from build123d import *

# Parameters (mm, degrees)
SKETCH1_R           = 12.2
BOSS_EXTRUDE1_DEPTH = 23.5
SKETCH2_R           = 12.5
BOSS_EXTRUDE2_DEPTH = 27
SKETCH3_R           = 3.5
BOSS_EXTRUDE3_DEPTH = 1.5
SKETCH4_R           = 2
BOSS_EXTRUDE4_DEPTH = 11


with BuildPart() as part:
    # Sketch1 → Boss-Extrude1 (new body, symmetric)
    with BuildSketch(Plane(origin=(0, 0, 0), x_dir=(1, 0, 0), z_dir=(0, 1, 0))):
        Circle(SKETCH1_R)
    extrude(amount=BOSS_EXTRUDE1_DEPTH, both=True)

    # Sketch2 → Boss-Extrude2 (add)
    with BuildSketch(Plane(origin=(0, 23.5, 0), x_dir=(1, 0, 0), z_dir=(0, 1, 0))):
        Circle(SKETCH2_R)
    extrude(amount=BOSS_EXTRUDE2_DEPTH)

    # Sketch3 → Boss-Extrude3 (add)
    with BuildSketch(Plane(origin=(0, 50.5, 0), x_dir=(1, 0, 0), z_dir=(0, 1, 0))):
        Circle(SKETCH3_R)
    extrude(amount=BOSS_EXTRUDE3_DEPTH)

    # Sketch4 → Boss-Extrude4 (add)
    with BuildSketch(Plane(origin=(0, 52, 0), x_dir=(1, 0, 0), z_dir=(0, 1, 0))):
        Circle(SKETCH4_R)
    extrude(amount=BOSS_EXTRUDE4_DEPTH)


solid = part.part
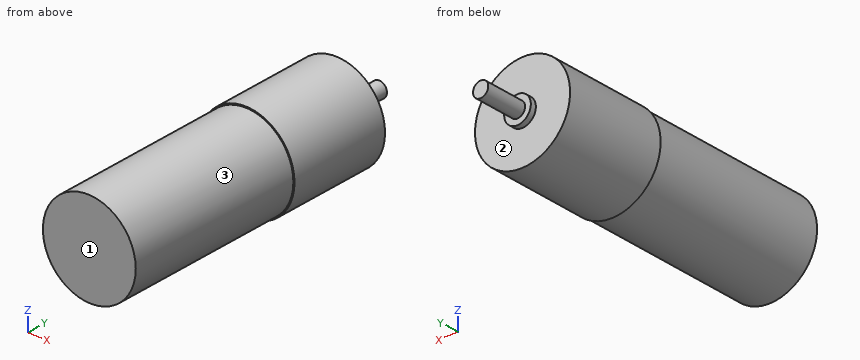
Geometry check sheet. Reference: the model listing, model coordinates, mm. Face numbers are marked on the shaded views. A direction names the side the tool comes from. Coordinates: 2 decimals unless noted, no trailing zeros. Order: outer loops, then holes, each group sorted by start corner. A loop starts at its lowest first (then second) coordinate and runs counter-clockwise, first axis right, second up. Notation, with made-up numbers: M 53,-0.5 L 107,-0.5 A29 ccw 107,32.5 Z; hole C -30,7 d7. An arc over 180 degrees is marked long. Use CSV: the item, a comma, the result in double quotes.
Item 1: Cross-section at B-B on z = 0. Record the cut outline in (x, y), then the cut area to 3 significant figures.
Returned:
outline,"M -12.5,23.5 L -12.2,23.5 L -12.2,-23.5 L 12.2,-23.5 L 12.2,23.5 L 12.5,23.5 L 12.5,50.5 L 3.5,50.5 L 3.5,52 L 2,52 L 2,63 L -2,63 L -2,52 L -3.5,52 L -3.5,50.5 L -12.5,50.5 Z"
area,"1,880 mm2"
Item 2: Cross-section at D-D on z = 10.25. Record the cut outline in (x, y).
Returned:
outline,"M -7.15,23.5 L -6.62,23.5 L -6.62,-23.5 L 6.62,-23.5 L 6.62,23.5 L 7.15,23.5 L 7.15,50.5 L -7.15,50.5 Z"
Item 3: Cross-section at A-A on x = 0. Record the cut outline in (y, z).
Returned:
outline,"M -23.5,-12.2 L 23.5,-12.2 L 23.5,-12.5 L 50.5,-12.5 L 50.5,-3.5 L 52,-3.5 L 52,-2 L 63,-2 L 63,2 L 52,2 L 52,3.5 L 50.5,3.5 L 50.5,12.5 L 23.5,12.5 L 23.5,12.2 L -23.5,12.2 Z"
Item 4: Thickness scan on line 1 along Y through (x, z) = (-7.25, -9.75); line 2 along Y through (x, z) = (2.5, -0.5); line 3 along X through (y, z) = (46.5, 0.5). Record the ranges inside material, lowest first.
Returned:
line 1,"y = -23.5 to 50.5"
line 2,"y = -23.5 to 52"
line 3,"x = -12.49 to 12.49"
Item 5: Cross-section at C-C on y = -4.5. Record the cut outline in (x, z).
Returned:
outline,"C 0,0 d24.4"
Item 6: Tool access check on the marked faces 1, 2 and 3. Record the directions out of +Z, -Z, +X, -X, +Y, -Y that give a thin tool (end or side, any length) a straight path to the whole face; none if there is none.
Returned:
face 1,"+Z, -Z, +X, -X, -Y"
face 2,"+Y"
face 3,"-Y"
Item 7: Gauge pin test, flat ends, axial feed: pin 1 Ø5 at (x, y) = (6.5, -6) entering from +Z; pin 2 Ø4 at (x, y) = (5, 43) entering from -Z; pin 3 Ø3 at (y, z) = (-12.5, -4) entering from +X. Record the tip position at first contact, or that the pin passes through.
Returned:
pin 1,"stops at z = 11.53"
pin 2,"stops at z = -12.13"
pin 3,"stops at x = 11.94"
